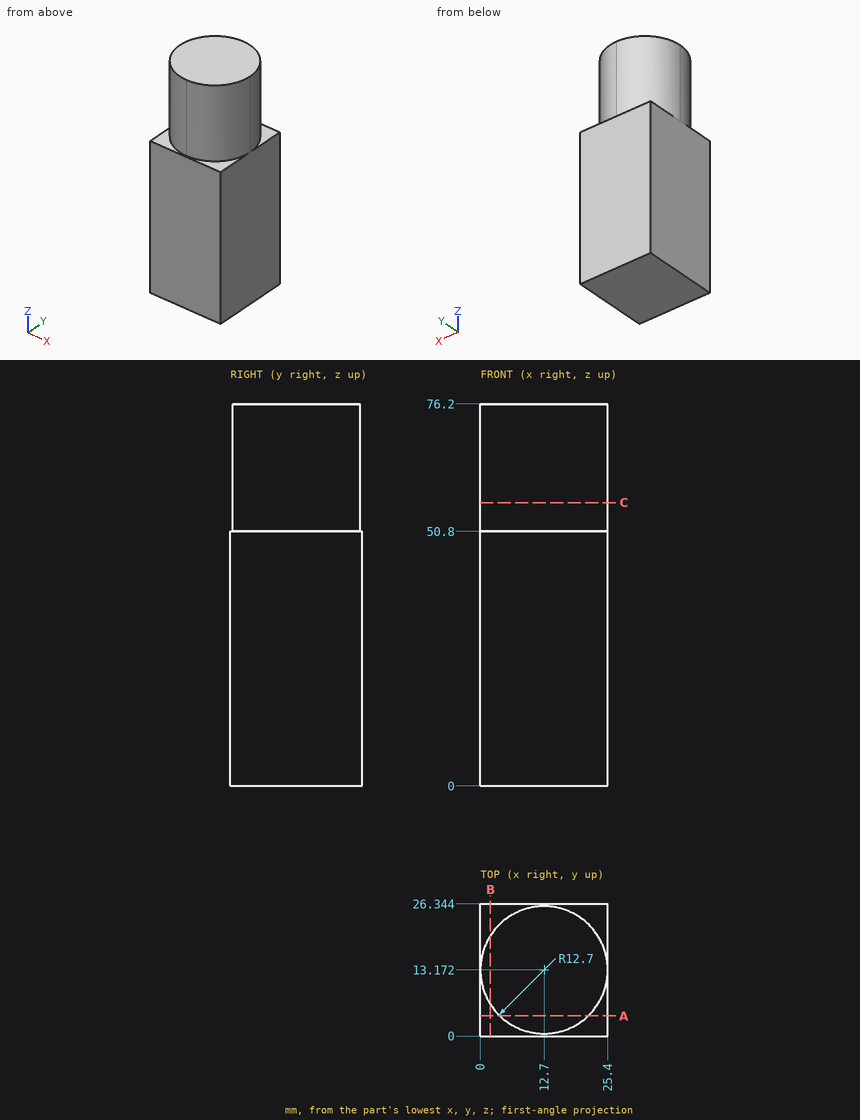
Answer from the drawing. Dimensions are ordinates in mm from the lowest x, y and z of the part. Give positions to 0.01 mm unless a question says otherwise; leave off trailing zeros. Write each loop counter-clockwise with the first axis right and the second up, starting at its lowest first coordinate (ties: lowest second). Pieces come first, ordered by that corner, then holes. Notation, with made-up numbers: (38, 47) - (48, 47) arc R7 cw to (48, 57) - close; hole circle Ø11 at (82, 50). An arc over 180 degrees is marked (long way). One line per item, written item: value. Start each with the question number.
1. Find section C-C (z = 56.5). Write down the section's boundary in (x, y), then the cut area to 3 significant figures.
2. Consider probe 1 along Z at (x, y) = (20.75, 2); probe 2 along X at (y, z) = (4.25, 55); probe 3 along Y at (x, z) = (6, 62.5). Determine where each line is inside the solid, lowest interval first.
3. Find section A-A (y = 4). Write down the section's boundary in (x, z) (1 decimal).
4. Find section B-B (x = 2). Write down the section's boundary in (y, z).
Geometry results:
1. outline: circle Ø25.4 at (12.7, 13.17)
1. area: 507 mm2
2. probe 1: 0 to 50.8
2. probe 2: 3.66 to 21.74
2. probe 3: 2.38 to 23.96
3. outline: (0, 0) - (25.4, 0) - (25.4, 50.8) - (21.5, 50.8) - (21.5, 76.2) - (3.9, 76.2) - (3.9, 50.8) - (0, 50.8) - close
4. outline: (0, 0) - (26.34, 0) - (26.34, 50.8) - (20.01, 50.8) - (20.01, 76.2) - (6.33, 76.2) - (6.33, 50.8) - (0, 50.8) - close
